```python
from build123d import *

# Parameters (mm, degrees)
SKETCH1_W                  = 93.1408
SKETCH1_H                  = 32.004
SKETCH2_R                  = 31.877
BOSS_EXTRUDE1_DEPTH        = 8.2296
SKETCH3_R                  = 15.0368
BOSS_EXTRUDE2_DEPTH        = 3.984
SKETCH4_R                  = 15.0368
BOSS_EXTRUDE3_DEPTH        = 1.016
BOSS_EXTRUDE3_TAPER        = 45
BOSS_EXTRUDE4_START        = 8.2296
SKETCH5_R                  = 31.877
BOSS_EXTRUDE4_DEPTH        = 8.2296
SKETCH6_R                  = 9.525
BOSS_EXTRUDE5_DEPTH        = 4
SKETCH7_R                  = 4
BOSS_EXTRUDE6_DEPTH        = 31.6
CUT_EXTRUDE1_REACH         = 125.971
CUT_EXTRUDE1_END_RADIUS    = 4
M3_5_CLEARANCE_HOLE1_D     = 4.0386
M3_5_CLEARANCE_HOLE1_DEPTH = 13.6144
M3_5_CLEARANCE_HOLE1_TIP   = 1.213317848
CHAMFER1_SIZE              = 1.016
CHAMFER2_SIZE              = 0.5
FILLET1_R                  = 1
CUT_EXTRUDE2_DEPTH         = 124.213928007
CUT_EXTRUDE2_DEPTH_BACK    = 124.213928007
SKETCH13_W                 = 12.7
SKETCH13_H                 = 41.153791371


with BuildPart() as part:
    # Sketch1 → Revolve1 (revolve)
    with BuildSketch(Plane.XY, mode=Mode.PRIVATE) as revolve1_sk:
        with Locations((54.8, 16.002)):
            Rectangle(SKETCH1_W, SKETCH1_H)
    revolve(revolve1_sk.sketch.rotate(Axis((8.2296, 0, 0), (1, 0, 0)), 270), axis=Axis((8.2296, 0, 0), (1, 0, 0)))

    # Sketch2 → Boss-Extrude1 (add)
    with BuildSketch(Plane(origin=(101.3704, 0, 0), x_dir=(0, 0, -1), z_dir=(1, 0, 0))):
        Circle(SKETCH2_R)
    extrude(amount=BOSS_EXTRUDE1_DEPTH)

    # Sketch3 → Boss-Extrude2 (add)
    with BuildSketch(Plane(origin=(109.6, 0, 0), x_dir=(0, 0, -1), z_dir=(1, 0, 0))):
        Circle(SKETCH3_R)
    extrude(amount=BOSS_EXTRUDE2_DEPTH)

    # Sketch4 → Boss-Extrude3 (add)
    with BuildSketch(Plane(origin=(113.584, 0, 0), x_dir=(0, 0, -1), z_dir=(1, 0, 0))):
        Circle(SKETCH4_R)
    extrude(amount=BOSS_EXTRUDE3_DEPTH, taper=BOSS_EXTRUDE3_TAPER)

    # Sketch5 → Boss-Extrude4 (add)
    with BuildSketch(Plane.ZY.offset(-8.2296).offset(BOSS_EXTRUDE4_START)):
        with Locations(Location((0, 0, 0), (0, 0, 180))):
            Circle(SKETCH5_R)
    extrude(amount=-BOSS_EXTRUDE4_DEPTH)

    # Sketch6 → Boss-Extrude5 (add)
    with BuildSketch(Plane.ZY):
        Circle(SKETCH6_R)
    extrude(amount=BOSS_EXTRUDE5_DEPTH)

    # Sketch7 → Boss-Extrude6 (add)
    with BuildSketch(Plane.ZY.offset(4)):
        Circle(SKETCH7_R)
    extrude(amount=BOSS_EXTRUDE6_DEPTH)

    # Cut-Extrude1: up to this cylinder (the profile starts inside it)
    cut_extrude1_end = Plane(origin=(-16.85, 0, 0), z_dir=(1, 0, 0)) * Cylinder(CUT_EXTRUDE1_END_RADIUS, 260.942, mode=Mode.PRIVATE)
    # Sketch8 → Cut-Extrude1 (cut, up to the surface)
    with BuildSketch(Plane.XZ.offset(-2.8), mode=Mode.PRIVATE) as cut_extrude1_sk1:
        with BuildLine():
            Line((-7.1, 1), (-26.6, 1))
            ThreePointArc((-26.6, 1), (-27.6, 0), (-26.6, -1))
            Line((-26.6, -1), (-7.1, -1))
            ThreePointArc((-7.1, -1), (-6.1, 0), (-7.1, 1))
        make_face()
    cut_extrude1_tool1 = extrude(cut_extrude1_sk1.sketch, amount=-CUT_EXTRUDE1_REACH, mode=Mode.PRIVATE) & cut_extrude1_end
    add(cut_extrude1_tool1.solids().sort_by_distance((-16.85, 2.8, 0))[0], mode=Mode.SUBTRACT)

    # Sketch9 → Revolve2 (revolve)
    with BuildSketch(Plane.XY.offset(-18.607090683), mode=Mode.PRIVATE) as revolve2_sk:
        Polygon((109.6, 15.525359639), (109.6, 11.207359639), (111.8479, 11.207359639), (111.8479, 13.325359639), (109.6479, 15.525359639), align=None)
    revolve(revolve2_sk.sketch.rotate(Axis((109.6, 11.207359639, -18.607090683), (1, 0, 0)), 270), axis=Axis((109.6, 11.207359639, -18.607090683), (1, 0, 0)))

    # Sketch10 → Revolve3 (revolve)
    with BuildSketch(Plane.XY.offset(-11.207359639), mode=Mode.PRIVATE) as revolve3_sk:
        Polygon((109.6, 22.925090683), (109.6, 18.607090683), (111.8479, 18.607090683), (111.8479, 20.725090683), (109.6479, 22.925090683), align=None)
    revolve(revolve3_sk.sketch.rotate(Axis((109.6, 18.607090683, -11.207359639), (1, 0, 0)), 270), axis=Axis((109.6, 18.607090683, -11.207359639), (1, 0, 0)))

    # M3.5 Clearance Hole1
    with Locations(Plane.ZY):
        with Locations((0, 25.4), (0, -25.4)):
            Hole(M3_5_CLEARANCE_HOLE1_D / 2, depth=M3_5_CLEARANCE_HOLE1_DEPTH)
            with Locations((0, 0, -(M3_5_CLEARANCE_HOLE1_DEPTH + M3_5_CLEARANCE_HOLE1_TIP / 2))):  # 118° drill point
                Cone(0, M3_5_CLEARANCE_HOLE1_D / 2, M3_5_CLEARANCE_HOLE1_TIP, mode=Mode.SUBTRACT)

    # Chamfer1
    chamfer1_edges = [part.edges().sort_by_distance(p)[0] for p in [
        (-4, 0, -9.525),
    ]]
    chamfer(chamfer1_edges, length=CHAMFER1_SIZE)

    # Chamfer2
    chamfer2_edges = [part.edges().sort_by_distance(p)[0] for p in [
        (-35.6, 0, -4),
    ]]
    chamfer(chamfer2_edges, length=CHAMFER2_SIZE)

    # Fillet1
    fillet1_edges = [part.edges().sort_by_distance(p)[0] for p in [
        (0, 0, 31.877),
        (109.6, 0, 31.877),
    ]]
    fillet(fillet1_edges, radius=FILLET1_R)

    # Sketch13 → Cut-Extrude2 (cut, two sides: drawn at the far end of the back side and taken through both)
    with BuildSketch(Plane(origin=(0, 0, 0), x_dir=(1, 0, 0), z_dir=(0, 1, 0)).offset(-CUT_EXTRUDE2_DEPTH_BACK)):
        with Locations((-29.25, 3.599946583)):
            Rectangle(SKETCH13_W, SKETCH13_H)
    extrude(amount=CUT_EXTRUDE2_DEPTH + CUT_EXTRUDE2_DEPTH_BACK, mode=Mode.SUBTRACT)


solid = part.part
```
For this review, take the finished solid that the model builds, in its own axes (mm). A direction names the side the tool comes from. Give positions to 0.01 mm unless a question says otherwise; leave off trailing zeros. Order: outer loops, then holes, each group sorted by start corner. A loop starts at its lowest first (then second) coordinate and runs counter-clockwise, first axis right, second up.
1) Wall thickness on line 1 (Y direction, x = 5.5, z = 0); line 2 (Y direction, x = 10, z = 0); line 3 (Z direction, x = 76.5, y = 8.5): over which ranges is each line inside the solid? List them lowest first.
2) For faces 1 (the face through (111.848, 19, -11)), 2 (the face through (-13.318, -3.905, -0.867)), 3 (the face through (109.6, -6, 14)), list the 3-axis set-ups (+Z, -Z, +X, -X, +Y, -Y) from which the entire face can be reached by the end or side of a thin tool; tool diameter is ignored.
3) Take a section at C-C (x = -13.5). Give the boundary of the cut face in (y, z), then the cut area to 3 significant figures.
4) Take a section at B-B (x = 10). Give the boundary of the cut face in (y, z), then the cut area to 3 significant figures.
5) Insertion check: pin 1 (0.9 mm diameter, centred on x = -13, y = 3.5, fed in from -Z); pin 2 (8 mm diameter, centred on y = 16.5, z = 16, fed in from -X); pin 3 (10 mm diameter, centred on x = 72.5, y = -23, fed in from +Z). Each pin has a flat end and moves straight along its axis. Give the tip position at first contact, or say it passes through.
6) Take a section at A-A (x = 87). Give the boundary of the cut face in (y, z).
7) The part is to be moulded in two halves that separate along Z. For faces 4 (the face through (114.6, 0, 0)), 5 (the face through (-1.471, -5.796, -7.559)), 6 (the face through (6.903, 27.402, 0.263)), say which applies: released by +Z, released by -Z, zero draft, split by the parting line, or undercut.
Derived:
1. line 1: y = -31.88 to -27.42, -23.38 to 23.38, 27.42 to 31.88
1. line 2: y = -32 to -27.42, -23.38 to 23.38, 27.42 to 32
1. line 3: z = -30.85 to 30.85
2. face 1: +Z, -Z, +X, +Y
2. face 2: -X
2. face 3: +X
3. outline: (2.8, -1) - (2.8, 1) - (3.87, 1) arc R4 ccw (long way) to (3.87, -1) - close
3. area: 47.9 mm2
4. outline: circle Ø64.01 at (0, 0); hole circle Ø4.04 at (-25.4, 0); hole circle Ø4.04 at (25.4, 0)
4. area: 3,190 mm2
5. pin 1: stops at z = -2.59
5. pin 2: stops at x = 0
5. pin 3: stops at z = 26.46
6. outline: circle Ø64.01 at (0, 0)
7. face 4: zero draft
7. face 5: split by the parting line
7. face 6: undercut
